Model file for the job. Use its own axes, mm. Face numbers are marked on the shaded views. A direction names the side the tool comes from. Give positions to 0.01 mm unless a question says otherwise; leave off trailing zeros. Loops run counter-clockwise (first coordinate to the right, second up) from the corner with the lowest first, then second, coordinate; pieces in that order, holes last. Notation, with made-up numbers: (51.25, 61) - (76.25, 61) arc R25 cw to (76.25, 85) - close; hole circle Ø6 at (89, 76.25). An arc over 180 degrees is marked (long way). Answer as CSV lines item,"result". Start each with the question number.
Item 1: Tool access for the marked faces 1 and 2: list every direction of +Z, -Z, +X, -X, +Y, -Y with a clear straight run to the whole face (end or side of a thin tool).
Item 2: Drill centre lines: L1, parallel to X at y = 91.5, z = 184.5; L2, parallel to X at y = 81.5, z = 359; L3, parallel to Z at x = 23, y = 86. Where is each one in solid material? Low to high. Write a range as from..to.
Item 3: Saw through at B-B on y = 18. Give the cut face in (x, z), plus the area to 3 significant figures.
Item 4: Pull direction X, two halves, no side cores. Call the marked faces 3, 4, 5 and 6: pulls with the +X half, pulls with the -X half, needs draft (parallel to the pull), parting line crosses it, or undercut.
Item 5: Saw through at A-A on z = 230. Give the cut face in (x, y), plus the area to 3 significant figures.
Item 6: Saw through at C-C on x = 33.5. Give the cut face in (y, z), plus the area to 3 significant figures.
Item 7: Pin check, flat tips, straight feed: pin 1 (19 mm diameter, centred on x = -22, y = 59.5, fed in from -Z); pin 2 (10 mm diameter, centred on x = -54.5, y = -34.5, fed in from +Z). Stop position of each tip, or through.
Item 8: Saw through at D-D on y = -50.8. Give the cut face in (x, z), plus the area to 3 significant figures.
from build123d import *

# Parameters (mm, degrees)
F0_W     = 254
F0_H     = 736.6
F0_W_2   = 203.2
F0_H_2   = 596.9
F0_W_3   = 127
F0_H_3   = 571.5
F0_W_4   = 101.6
F0_H_4   = 546.1
F0_H_5   = 63.5
F1_DEPTH = 127
F2_DEPTH = 25.4
F3_DEPTH = 88.9
F4_R     = 50.79999
F5_DEPTH = 76.2
F6_R     = 19.05
F7_DEPTH = 38.1


# Not quite as in the source:
# - a fillet or chamfer is up to 0.001 mm smaller than in the source, because OpenCascade refuses the exact size
# - a feature names something its author has since deleted; it is built from what else it names


with BuildPart() as f1:
    # F0 (on Front) → F1 (new body)
    with BuildSketch(Plane.XZ):
        with Locations((0, 241.3)):
            Rectangle(F0_W, F0_H)
        with Locations((0, 298.45)):
            Rectangle(F0_W_2, F0_H_2, mode=Mode.SUBTRACT)
        with Locations((0, 298.45)):
            Rectangle(F0_W_2, F0_H_2)
        with Locations((0, 296.15)):
            Rectangle(F0_W_3, F0_H_3, mode=Mode.SUBTRACT)
        with Locations((0, 296.15)):
            Rectangle(F0_W_3, F0_H_3)
        with Locations((0, 293.85)):
            Rectangle(F0_W_4, F0_H_4, mode=Mode.SUBTRACT)
        with Locations((0, -158.75)):
            Rectangle(F0_W, F0_H_5)
    extrude(amount=-F1_DEPTH)

    # F0 (on Front) → F2 (cut)
    with BuildSketch(Plane.XZ):
        with Locations((0, 298.45)):
            Rectangle(F0_W_2, F0_H_2)
        with Locations((0, 296.15)):
            Rectangle(F0_W_3, F0_H_3, mode=Mode.SUBTRACT)
    extrude(amount=-F2_DEPTH, mode=Mode.SUBTRACT)

    # F0 (on Front) → F3 (cut)
    with BuildSketch(Plane.XZ):
        with Locations((0, 296.15)):
            Rectangle(F0_W_3, F0_H_3)
        with Locations((0, 293.85)):
            Rectangle(F0_W_4, F0_H_4, mode=Mode.SUBTRACT)
    extrude(amount=-F3_DEPTH, mode=Mode.SUBTRACT)

    # F4 (radius 50.8 in the source; OpenCascade refuses exactly that, so slightly less here)
    f4_edges = [f1.edges().sort_by_distance(p)[0] for p in [
        (50.8, 107.95, 566.9),
        (-50.8, 107.95, 566.9),
        (-50.8, 107.95, 20.8),
        (50.8, 107.95, 20.8),
    ]]
    fillet(f4_edges, radius=F4_R)

    # F0 (on Front) → F5 (join)
    with BuildSketch(Plane.XZ):
        with Locations((0, -158.75)):
            Rectangle(F0_W, F0_H_5)
    extrude(amount=F5_DEPTH)

    # F6 (on face) → F7 (join)
    with BuildSketch(Plane(origin=(0, 0, -190.5), x_dir=(1, 0, 0), z_dir=(0, 0, -1))):
        with Locations((-101.6, 50.8)):
            Circle(F6_R)
        with Locations((101.6, 50.8)):
            Circle(F6_R)
        with Locations((-101.6, -101.6)):
            Circle(F6_R)
        with Locations((101.6, -101.6)):
            Circle(F6_R)
    extrude(amount=F7_DEPTH)


solid = f1.part
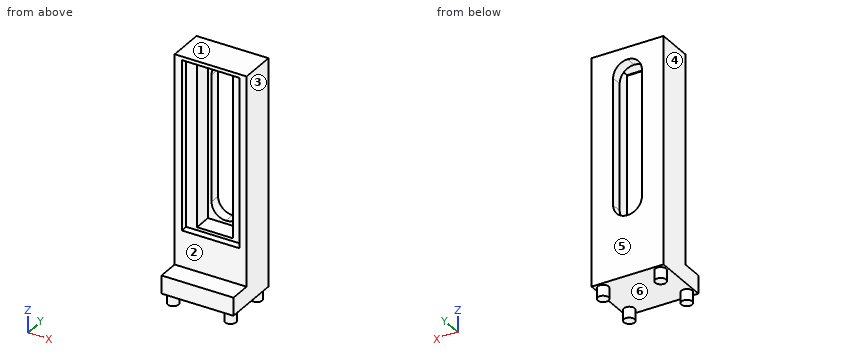
Responses:
1,face 1,"+Z, +X, -X, +Y, -Y"
1,face 2,"+Z, +X, -X, -Y"
2,L1,"-127..-50.8, 50.8..127"
2,L2,"-127..-63.5, 63.5..127"
2,L3,"-190.5..10.4, 581.9..609.6"
3,outline,"(-127, -190.5) - (127, -190.5) - (127, 609.6) - (-127, 609.6) - close; hole (-101.6, 0) - (101.6, 0) - (101.6, 596.9) - (-101.6, 596.9) - close"
3,area,"81,900 mm2"
4,face 3,"pulls with the +X half"
4,face 4,"pulls with the -X half"
4,face 5,"needs draft"
4,face 6,"undercut"
5,outline,"(-127, 0) - (-101.6, 0) - (-101.6, 25.4) - (-63.5, 25.4) - (-63.5, 88.9) - (-50.8, 88.9) - (-50.8, 127) - (-127, 127) - close; (50.8, 88.9) - (63.5, 88.9) - (63.5, 25.4) - (101.6, 25.4) - (101.6, 0) - (127, 0) - (127, 127) - (50.8, 127) - close"
5,area,"15,200 mm2"
6,outline,"(-76.2, -190.5) - (127, -190.5) - (127, 33.41) - (88.9, 33.41) - (88.9, 10.4) - (25.4, 10.4) - (25.4, 0) - (0, 0) - (0, -127) - (-76.2, -127) - close; (0, 596.9) - (25.4, 596.9) - (25.4, 581.9) - (88.9, 581.9) - (88.9, 554.29) - (127, 554.29) - (127, 609.6) - (0, 609.6) - close"
6,area,"35,200 mm2"
7,pin 1,"z = -190.5"
7,pin 2,"z = -127"
8,outline,"(-127, -190.5) - (-120.65, -190.5) - (-120.65, -228.6) - (-82.55, -228.6) - (-82.55, -190.5) - (82.55, -190.5) - (82.55, -228.6) - (120.65, -228.6) - (120.65, -190.5) - (127, -190.5) - (127, -127) - (-127, -127) - close"
8,area,"19,000 mm2"
